Input: part model. Units: mm. Frame: model coordinates. Give positions to 0.01 mm unless a question says otherwise; leave off trailing zeros. Write each loop counter-clockwise with the first axis right and the second up, starting at its lowest first coordinate (ties: lowest second). Pieces come first, ordered by that corner, then holes. Notation, with made-up numbers: (3, 82) - (53, 82) arc R12 ccw to (53, 92) - close; hole circle Ø1 at (42, 5.5). An arc over 180 degrees is marked (long way). Use a Markdown table: item, result. Add a question column.
1. Section query C-C, the plane z = -28. Return loops of the section in (x, y), plus the area to 3 significant figures.
2. Material intervals for probe 1 along X at (y, z) = (1.4, 0); probe 2 along Z at (x, y) = (-78, 1.55); probe 3 along Z at (x, y) = (-36, 1.45), sorted ascending.
3. Section query A-A, the plane x = -45. Return loops of the section in (y, z).
4. Section query D-D, the plane y = 0.65. Count the separate pieces of the cut face and the enclosed holes in it, plus the area to 3 significant figures.
5. Pin query (flat end, axial travel): pin 1 (1.5 mm diameter, centred on x = -61.5, y = 2.5, fed in from +Z). Return the tip coordinate at first contact, or that it passes through.
6. Section query B-B, the plane x = -7.5. Return loops of the section in (y, z).
```python
from build123d import *

# Parameters (mm, degrees)
BOSS_EXTRUDE1_DEPTH                    = 3.18
BOSS_EXTRUDE2_DEPTH                    = 3.18
FILLET1_R                              = 3
SKETCH3_R                              = 1.5
CUT_EXTRUDE1_DEPTH                     = 3.18
CIRPATTERN1_COUNT                      = 3
CIRPATTERN1_ANGLE                      = 72
FILLET1_OF_CIRPATTERN1_R               = 3
CIRPATTERN1_THE_OTHER_WAY_COUNT        = 3
CIRPATTERN1_THE_OTHER_WAY_ANGLE        = 72
FILLET1_OF_CIRPATTERN1_THE_OTHER_WAY_R = 3
CHAMFER1_SIZE                          = 1


with BuildPart() as part:
    # Sketch1 → Boss-Extrude1 (new body)
    with BuildSketch(Plane(origin=(0, 0, 0), x_dir=(1, 0, 0), z_dir=(0, 1, 0))):
        with BuildLine():
            Line((0, 103), (0, 97))
            ThreePointArc((0, 97), (-97, 0), (0, -97))
            Line((0, -97), (0, -103))
            ThreePointArc((0, -103), (-103, 0), (0, 103))
        make_face()
    extrude(amount=BOSS_EXTRUDE1_DEPTH)

    # Sketch2 → Boss-Extrude2 (add)
    with BuildSketch(Plane(origin=(0, 3.18, 0), x_dir=(1, 0, 0), z_dir=(0, 1, 0))):
        with BuildLine():
            ThreePointArc((-97.965532202, 1.858929465), (-97.515712838, 2.43334932), (-96.956578947, 2.902033567))
            ThreePointArc((-96.956578947, 2.902033567), (-96.947168056, 3.201032006), (-96.936835104, 3.5))
            Line((-96.936835104, 3.5), (-97.965532202, 1.858929465))
        make_face()
        with BuildLine():
            ThreePointArc((-96.956578947, 2.902033567), (-96.022957115, 3.347171753), (-95, 3.5))
            Line((-95, 3.5), (-96.936835104, 3.5))
            ThreePointArc((-96.936835104, 3.5), (-96.947168056, 3.201032006), (-96.956578947, 2.902033567))
        make_face()
        with BuildLine():
            Line((-97.965532202, -1.858929465), (-96.936835104, -3.5))
            ThreePointArc((-96.936835104, -3.5), (-96.947168056, -3.201032006), (-96.956578947, -2.902033567))
            ThreePointArc((-96.956578947, -2.902033567), (-97.515712838, -2.43334932), (-97.965532202, -1.858929465))
        make_face()
        with BuildLine():
            Line((-96.936835104, -3.5), (-95, -3.5))
            ThreePointArc((-95, -3.5), (-96.022957115, -3.347171753), (-96.956578947, -2.902033567))
            ThreePointArc((-96.956578947, -2.902033567), (-96.947168056, -3.201032006), (-96.936835104, -3.5))
        make_face()
        with BuildLine():
            ThreePointArc((-96.956578947, -2.902033567), (-96.022957115, -3.347171753), (-95, -3.5))
            ThreePointArc((-95, -3.5), (-92.525126266, -2.474873734), (-91.5, 0))
            ThreePointArc((-91.5, 0), (-92.525126266, 2.474873734), (-95, 3.5))
            ThreePointArc((-95, 3.5), (-96.022957115, 3.347171753), (-96.956578947, 2.902033567))
            ThreePointArc((-96.956578947, 2.902033567), (-97, 0), (-96.956578947, -2.902033567))
        make_face()
        with BuildLine():
            ThreePointArc((-97.965532202, -1.858929465), (-97.515712838, -2.43334932), (-96.956578947, -2.902033567))
            ThreePointArc((-96.956578947, -2.902033567), (-97, 0), (-96.956578947, 2.902033567))
            ThreePointArc((-96.956578947, 2.902033567), (-97.515712838, 2.43334932), (-97.965532202, 1.858929465))
            ThreePointArc((-97.965532202, 1.858929465), (-98.5, 0), (-97.965532202, -1.858929465))
        make_face()
    boss_extrude2 = extrude(amount=-BOSS_EXTRUDE2_DEPTH)

    # Fillet1
    fillet1_edges = [part.edges().sort_by_distance(p)[0] for p in [
        (-96.936835104, 1.59, -3.5),
        (-96.936835104, 1.59, 3.5),
    ]]
    fillet(fillet1_edges, radius=FILLET1_R)

    # Sketch3 → Cut-Extrude1 (cut)
    with BuildSketch(Plane(origin=(0, 3.18, 0), x_dir=(1, 0, 0), z_dir=(0, 1, 0))):
        with Locations((-95, 0)):
            Circle(SKETCH3_R)
    cut_extrude1 = extrude(amount=-CUT_EXTRUDE1_DEPTH, mode=Mode.SUBTRACT)

    # CirPattern1: Boss-Extrude2, Cut-Extrude1 ×3 about axis
    cirpattern1_axis = Axis((0, 0, 0), (0, -1, 0))
    for i in range(1, CIRPATTERN1_COUNT):
        add(boss_extrude2.rotate(cirpattern1_axis, i * CIRPATTERN1_ANGLE / (CIRPATTERN1_COUNT - 1)))
        add(cut_extrude1.rotate(cirpattern1_axis, i * CIRPATTERN1_ANGLE / (CIRPATTERN1_COUNT - 1)), mode=Mode.SUBTRACT)

    # Fillet1 of CirPattern1
    fillet1_of_cirpattern1_edges = [part.edges().sort_by_distance(p)[0] for p in [
        (-76.366298597, 1.59, -59.809601558),
        (-80.480795363, 1.59, -54.146482598),
        (-26.626431621, 1.59, -93.273968175),
        (-33.283827235, 1.59, -91.110849214),
    ]]
    fillet(fillet1_of_cirpattern1_edges, radius=FILLET1_OF_CIRPATTERN1_R)

    # CirPattern1 the other way: Boss-Extrude2, Cut-Extrude1 ×3 about axis
    cirpattern1_the_other_way_axis = Axis((0, 0, 0), (0, 1, 0))
    for i in range(1, CIRPATTERN1_THE_OTHER_WAY_COUNT):
        add(boss_extrude2.rotate(cirpattern1_the_other_way_axis, i * CIRPATTERN1_THE_OTHER_WAY_ANGLE / (CIRPATTERN1_THE_OTHER_WAY_COUNT - 1)))
        add(cut_extrude1.rotate(cirpattern1_the_other_way_axis, i * CIRPATTERN1_THE_OTHER_WAY_ANGLE / (CIRPATTERN1_THE_OTHER_WAY_COUNT - 1)), mode=Mode.SUBTRACT)

    # Fillet1 of CirPattern1 the other way
    fillet1_of_cirpattern1_the_other_way_edges = [part.edges().sort_by_distance(p)[0] for p in [
        (-80.480795363, 1.59, 54.146482598),
        (-76.366298597, 1.59, 59.809601558),
        (-33.283827235, 1.59, 91.110849214),
        (-26.626431621, 1.59, 93.273968175),
    ]]
    fillet(fillet1_of_cirpattern1_the_other_way_edges, radius=FILLET1_OF_CIRPATTERN1_THE_OTHER_WAY_R)

    # Chamfer1
    chamfer1_edges = [part.edges().sort_by_distance(p)[0] for p in [
        (0, 3.18, -100),
        (0, 3.18, 100),
    ]]
    chamfer(chamfer1_edges, length=CHAMFER1_SIZE)


solid = part.part
```
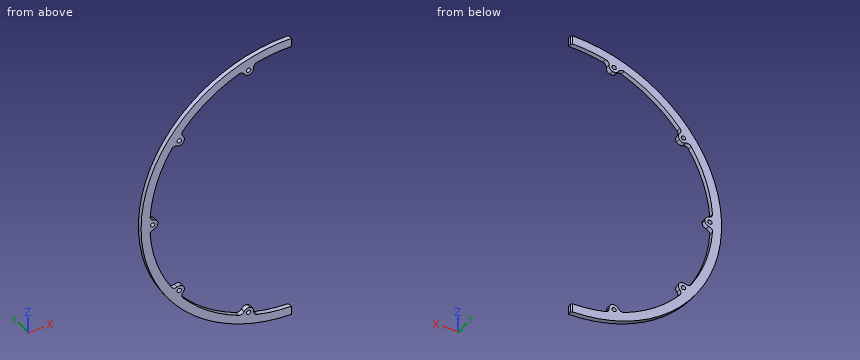
Result sheet:
| question | item | result |
|---|---|---|
| 1 | outline | (-99.12, 0) - (-92.87, 0) - (-92.87, 3.18) - (-99.12, 3.18) - close |
| 1 | area | 19.9 mm² |
| 2 | probe 1 | x = -103 to -96.5, -93.5 to -91.5 |
| 2 | probe 2 | z = -67.27 to -56.81, -54.87 to -52.53, 52.53 to 54.87, 56.81 to 67.27 |
| 2 | probe 3 | z = -96.5 to -90.07, 90.07 to 96.5 |
| 3 | outline | (0, -92.65) - (3.18, -92.65) - (3.18, -85.93) - (0, -85.93) - close; (0, 85.93) - (3.18, 85.93) - (3.18, 92.65) - (0, 92.65) - close |
| 4 | separate pieces | 1 |
| 4 | enclosed holes | 5 |
| 4 | area | 2,030 mm² |
| 5 | pin 1 | stops at z = 83.18 |
| 6 | outline | (0, -102.73) - (3.18, -102.73) - (3.18, -96.71) - (0, -96.71) - close; (0, 96.71) - (3.18, 96.71) - (3.18, 102.73) - (0, 102.73) - close |
